```python
from build123d import *

# Parameters (mm, degrees)
BOSS_EXTRUDE1_DEPTH = 76.2
FILLET1_R           = 25.4
SKETCH2_R           = 12.7
CUT_EXTRUDE1_DEPTH  = 252.476
SKETCH7_R           = 6.35


with BuildPart() as part:
    # Sketch1 → Boss-Extrude1 (new body)
    with BuildSketch(Plane.XY):
        Polygon((0, 0), (50.8, 0), (50.8, 101.6), (25.4, 101.6), (25.4, 50.8), (0, 25.4), align=None)
    extrude(amount=BOSS_EXTRUDE1_DEPTH)

    # Fillet1
    fillet1_edges = [part.edges().sort_by_distance(p)[0] for p in [
        (38.1, 101.6, 76.2),
    ]]
    fillet(fillet1_edges, radius=FILLET1_R)

    # Sketch2 → Cut-Extrude1 (cut, symmetric)
    with BuildSketch(Plane(origin=(0, 0, 0), x_dir=(0, 0, -1), z_dir=(1, 0, 0))):
        with Locations((-38.1, 76.2)):
            Circle(SKETCH2_R)
    extrude(amount=CUT_EXTRUDE1_DEPTH, both=True, mode=Mode.SUBTRACT)

    # Cut-Sweep1: sweep along a path in Sketch4
    with BuildLine(Plane(origin=(38.1, 0, -38.1), x_dir=(0, 0, 1), z_dir=(-1, 0, 0))) as cut_sweep1_path:
        Line((76.2, 76.2), (106.860512242, 94.160512242))
    # Sketch7 → Cut-Sweep1 (sweep, cut)
    with BuildSketch(Plane(origin=(38.1, 94.160512242, 68.760512242), x_dir=(1, 0, 0), z_dir=(0, 0.7071067811865479, 0.7071067811865472))):
        Circle(SKETCH7_R)
    sweep(path=cut_sweep1_path.line, mode=Mode.SUBTRACT)


solid = part.part
```
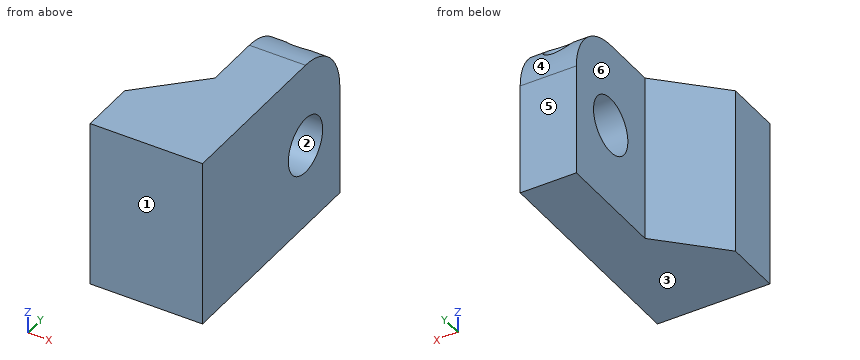
Here's how the part is built. I have some questions about the finished solid (model axes, mm). Face numbers are marked on the shaded views. A direction names the side the tool comes from. Coordinates: 2 decimals unless noted, no trailing zeros. Order: outer loops, then holes, each group sorted by start corner. A loop starts at its lowest first (then second) coordinate and runs counter-clockwise, first axis right, second up. Notation, with made-up numbers: (46.25, 82.25) - (58.25, 82.25) arc R22 ccw to (58.25, 104.25) - close; hole circle Ø11 at (-27, 39.5). An arc over 180 degrees is marked (long way). One line per question, with ' | ' between items. Start each with the question number.
1. I'm going to push flat-ended pins straight in: pin 1 Ø15 at (y, z) = (76.2, 38.1) entering from +X; pin 2 Ø10 at (x, z) = (39, 66.5) entering from +Y. Where does each tip first touch, or does it pass through?
2. If we section it at B-B (y = 73): Write out the boundary of the cut face in (x, z), and give its area (3 significant figures).
3. If we section it at A-A (z = 38.1): Write out the boundary of the cut face in (x, y).
4. Which directions (+Z, -Z, +X, -X, +Y, -Y) give clear straight access to the entire face, cutting with the end or side of a thin tool? Please do the marked faces 5 and 6.
5. If we section it at C-C (y = 34): Write out the boundary of the cut face in (x, z), and give its area (3 significant figures).
6. Please list where these lines run through material, in increasing order: line 1 along Y through (x, z) = (39, 38); line 2 along Z through (x, y) = (39, 76); line 3 along X through (y, z) = (54, 65.5). Write a range as [from, to].
7. If we mould it in two halves opening along Z, with no side actions, what happens to the marked faces 1, 2, 3 and 4? For each: released by +Z, released by -Z, zero draft, split by the parting line, or undercut.
Model answer:
1) pin 1: passes through | pin 2: stops at y = 99.24
2) outline: (25.4, 0) - (50.8, 0) - (50.8, 25.81) - (25.4, 25.81) - close; (25.4, 50.39) - (50.8, 50.39) - (50.8, 76.2) - (25.4, 76.2) - close | area: 1,310 mm²
3) outline: (0, 0) - (50.8, 0) - (50.8, 63.5) - (25.4, 63.5) - (25.4, 50.8) - (0, 25.4) - close; (25.4, 88.9) - (50.8, 88.9) - (50.8, 101.6) - (25.4, 101.6) - close
4) face 5: +Z, -Z, +X, -X, +Y | face 6: +Z, -Z, -X, +Y
5) outline: (8.6, 0) - (50.8, 0) - (50.8, 76.2) - (8.6, 76.2) - close | area: 3,220 mm²
6) line 1: y = [0, 63.5], [88.9, 101.6] | line 2: z = [0, 25.4], [50.8, 76.2] | line 3: x = [25.4, 50.8]
7) face 1: zero draft | face 2: undercut | face 3: released by -Z | face 4: released by +Z
